The listing builds one solid part. Answer for the finished solid, in the listing's coordinates (mm). A direction names the side the tool comes from. Round coordinates to 2 decimals unless told otherwise and drop trailing zeros. Order: outer loops, then holes, each group sorted by start corner. A loop starts at its lowest first (then second) coordinate and runs counter-clockwise, first axis right, second up. Notation, with made-up numbers: (26, 59.5) -> (46, 59.5) arc R15 cw to (46, 69.5) -> close; hole circle Ø9 at (57.25, -11.5). An arc over 180 degrees is marked (long way). Answer in a Markdown table with one row per item. Add a question column.
Solid Edge part; units mm, degrees
sketch "Sketch1" plane through (0, 0, 0) normal (0, 0, 1) x (1, 0, 0)
  line L0 (0, 32.5628) -> (110, 32.5628)
  line L1 (110, 32.5628) -> (110, -77.4372)
  line L2 (110, -77.4372) -> (0, -77.4372)
  line L3 (0, 32.5628) -> (0, -77.4372)
extrude "Protrusion1" add sketch "Sketch1" along normal blind 27
sketch "Sketch2" plane through (55, -22.4372, 27) normal (0, 0, 1) x (1, 0, 0)
  line L0 (-53, -53) -> (53, -53)
  line L1 (53, -53) -> (53, 53)
  line L2 (53, 53) -> (-53, 53)
  line L3 (-53, 53) -> (-53, -53)
extrude "ExtrudedCutout_1" cut sketch "Sketch2" against normal blind 25
sketch "Sketch3" plane through (55, 30.5628, 14.5) normal (0, -1, 0) x (1, 0, 0)
  circle A0 centre (-18.3168, -3.0528) radius 6
extrude "ExtrudedCutout_2" cut sketch "Sketch3" against normal blind 2
sketch "Sketch4" plane through (110, -22.4372, 13.5) normal (1, 0, 0) x (0, 1, 0)
  line L0 (23.663, -1.8749) -> (45.663, -1.8749)
  line L1 (45.663, -1.8749) -> (45.663, 3.8251)
  line L2 (45.663, 3.8251) -> (23.663, 3.8251)
  line L3 (23.663, 3.8251) -> (23.663, -1.8749)
extrude "ExtrudedCutout_3" cut sketch "Sketch4" against normal blind 2
sketch "Sketch5" plane through (108, -22.4372, 14.5) normal (-1, 0, 0) x (0, 0, 1)
  line L0 (2.8251, 47.663) -> (4.8251, 47.663)
  line L1 (4.8251, 47.663) -> (4.8251, 21.663)
  line L2 (4.8251, 21.663) -> (-4.8749, 21.663)
  line L3 (-4.8749, 21.663) -> (-4.8749, 47.663)
  line L4 (-4.8749, 47.663) -> (2.8251, 47.663)
extrude "ExtrudedProtrusion_2" add sketch "Sketch5" along normal blind 7.2
sketch "Sketch6" plane through (110, -22.4372, 13.5) normal (1, 0, 0) x (0, 1, 0)
  line L0 (23.663, 3.8251) -> (45.663, 3.8251)
  line L1 (45.663, 3.8251) -> (45.663, -1.8749)
  line L2 (45.663, -1.8749) -> (23.663, -1.8749)
  line L3 (23.663, -1.8749) -> (23.663, 3.8251)
extrude "ExtrudedCutout_4" cut sketch "Sketch6" against normal blind 7
sketch "Sketch7" plane through (100.8, 12.2258, 14.4751) normal (-1, 0, 0) x (0, -1, 0)
  line L0 (0, -1.85) -> (9, -1.85)
  line L1 (9, -1.85) -> (9, 1.85)
  line L2 (9, 1.85) -> (-9, 1.85)
  line L3 (-9, 1.85) -> (-9, -1.85)
  line L4 (-9, -1.85) -> (0, -1.85)
extrude "ExtrudedCutout_5" cut sketch "Sketch7" against normal blind 26.8721
sketch "Sketch8" plane through (110, -22.4372, 13.5) normal (1, 0, 0) x (0, 1, 0)
  line L0 (8.2756, -1.8749) -> (17.2756, -1.8749)
  line L1 (17.2756, -1.8749) -> (17.2756, 3.8251)
  line L2 (17.2756, 3.8251) -> (8.2756, 3.8251)
  line L3 (8.2756, 3.8251) -> (8.2756, -1.8749)
extrude "ExtrudedCutout_6" cut sketch "Sketch8" against normal blind 30.5101
sketch "Sketch9" plane through (108, -22.4372, 14.5) normal (-1, 0, 0) x (0, -1, 0)
  line L0 (-17.2756, 4.8251) -> (-6.2756, 4.8251)
  line L1 (-6.2756, 4.8251) -> (-6.2756, -4.8749)
  line L2 (-6.2756, -4.8749) -> (-19.2756, -4.8749)
  line L3 (-19.2756, -4.8749) -> (-19.2756, 4.8251)
  line L4 (-19.2756, 4.8251) -> (-17.2756, 4.8251)
extrude "ExtrudedProtrusion_3" add sketch "Sketch9" along normal blind 7.2
sketch "Sketch10" plane through (108, -9.6616, 14.4751) normal (1, 0, 0) x (0, 1, 0)
  line L0 (-2.5, -1.85) -> (0, -1.85)
  line L1 (0, -1.85) -> (2.5, -1.85)
  line L2 (2.5, -1.85) -> (2.5, 1.85)
  line L3 (2.5, 1.85) -> (-2.5, 1.85)
  line L4 (-2.5, 1.85) -> (-2.5, -1.85)
extrude "ExtrudedCutout_8" cut sketch "Sketch10" against normal blind 9.4627
sketch "Sketch11" plane through (108, -9.6616, 14.4751) normal (1, 0, 0) x (0, 1, 0)
  line L0 (-4.5, 2.85) -> (4.5, 2.85)
  line L1 (4.5, 2.85) -> (4.5, -2.85)
  line L2 (4.5, -2.85) -> (-4.5, -2.85)
  line L3 (-4.5, -2.85) -> (-4.5, 2.85)
extrude "ExtrudedCutout_10" cut sketch "Sketch11" against normal blind 7
sketch "Sketch12" plane through (0, -22.4372, 13.5) normal (-1, 0, 0) x (0, -1, 0)
  line L0 (-45.663, 3.8251) -> (-45.663, -1.8749)
  line L1 (-45.663, -1.8749) -> (-25.663, -1.8749)
  line L2 (-25.663, -1.8749) -> (-25.663, 3.8251)
  line L3 (-25.663, 3.8251) -> (-45.663, 3.8251)
extrude "ExtrudedCutout_11" cut sketch "Sketch12" against normal blind 2
sketch "Sketch13" plane through (2, -22.4372, 14.5) normal (1, 0, 0) x (0, 0, -1)
  line L0 (4.8749, 23.663) -> (-4.8251, 23.663)
  line L1 (-4.8251, 23.663) -> (-4.8251, 47.663)
  line L2 (-4.8251, 47.663) -> (4.8749, 47.663)
  line L3 (4.8749, 47.663) -> (4.8749, 23.663)
extrude "ExtrudedProtrusion_4" add sketch "Sketch13" along normal blind 7.2
sketch "Sketch14" plane through (0, -22.4372, 13.5) normal (-1, 0, 0) x (0, -1, 0)
  line L0 (-45.663, -1.8749) -> (-45.663, 3.8251)
  line L1 (-45.663, 3.8251) -> (-25.663, 3.8251)
  line L2 (-25.663, 3.8251) -> (-25.663, -1.8749)
  line L3 (-25.663, -1.8749) -> (-45.663, -1.8749)
extrude "ExtrudedCutout_12" cut sketch "Sketch14" against normal blind 7
sketch "Sketch15" plane through (7, 13.2258, 14.4751) normal (-1, 0, 0) x (0, 0, 1)
  line L0 (1.85, 8) -> (-1.85, 8)
  line L1 (-1.85, 8) -> (-1.85, -8)
  line L2 (-1.85, -8) -> (1.85, -8)
  line L3 (1.85, -8) -> (1.85, 8)
extrude "Cutout1" cut sketch "Sketch15" against normal blind 13.8716
sketch "Sketch16" plane through (2, -22.4372, 14.5) normal (1, 0, 0) x (0, 0, -1)
  line L0 (-4.8251, 19.2756) -> (4.8749, 19.2756)
  line L1 (4.8749, 19.2756) -> (4.8749, 6.2756)
  line L2 (4.8749, 6.2756) -> (-4.8251, 6.2756)
  line L3 (-4.8251, 6.2756) -> (-4.8251, 19.2756)
extrude "ExtrudedProtrusion_7" add sketch "Sketch16" along normal blind 7.2
sketch "Sketch17" plane through (9.2, -9.6616, 14.4751) normal (1, 0, 0) x (0, 0, -1)
  line L0 (-1.85, 2.5) -> (1.85, 2.5)
  line L1 (1.85, 2.5) -> (1.85, -2.5)
  line L2 (1.85, -2.5) -> (-1.85, -2.5)
  line L3 (-1.85, -2.5) -> (-1.85, 2.5)
extrude "ExtrudedCutout_16" cut sketch "Sketch17" against normal blind 15.454
sketch "Sketch18" plane through (0, -22.4372, 13.5) normal (-1, 0, 0) x (0, 0, 1)
  line L0 (-1.8749, 17.2756) -> (3.8251, 17.2756)
  line L1 (3.8251, 17.2756) -> (3.8251, 8.2756)
  line L2 (3.8251, 8.2756) -> (-1.8749, 8.2756)
  line L3 (-1.8749, 8.2756) -> (-1.8749, 17.2756)
extrude "ExtrudedCutout_17" cut sketch "Sketch18" against normal blind 7
sketch "Sketch19" plane through (2, -22.4372, 14.5) normal (1, 0, 0) x (0, 0, -1)
  line L0 (-4.8251, 1.8941) -> (4.8749, 1.8941)
  line L1 (4.8749, 1.8941) -> (4.8749, -11.1059)
  line L2 (4.8749, -11.1059) -> (-4.8251, -11.1059)
  line L3 (-4.8251, -11.1059) -> (-4.8251, 1.8941)
extrude "ExtrudedProtrusion_8" add sketch "Sketch19" along normal blind 7.2
sketch "Sketch20" plane through (9.2, -27.0431, 14.4751) normal (1, 0, 0) x (0, 0, -1)
  line L0 (-1.85, 2.5) -> (-1.85, -2.5)
  line L1 (-1.85, -2.5) -> (1.85, -2.5)
  line L2 (1.85, -2.5) -> (1.85, 2.5)
  line L3 (1.85, 2.5) -> (-1.85, 2.5)
extrude "ExtrudedCutout_18" cut sketch "Sketch20" against normal blind 324.0976
sketch "Sketch21" plane through (0, -22.4372, 13.5) normal (-1, 0, 0) x (0, 0, 1)
  line L0 (-1.8749, -0.1059) -> (3.8251, -0.1059)
  line L1 (3.8251, -0.1059) -> (3.8251, -9.1059)
  line L2 (3.8251, -9.1059) -> (-1.8749, -9.1059)
  line L3 (-1.8749, -9.1059) -> (-1.8749, -0.1059)
extrude "ExtrudedCutout_19" cut sketch "Sketch21" against normal blind 7
sketch "Sketch22" plane through (55, -22.4372, 27) normal (0, 0, 1) x (1, 0, 0)
  line L0 (-55, 55) -> (55, 55)
  line L1 (55, 55) -> (55, -55)
  line L2 (55, -55) -> (-55, -55)
  line L3 (-55, -55) -> (-55, 55)
extrude "ExtrudedProtrusion_9" add sketch "Sketch22" along normal blind 35
sketch "Sketch23" plane through (55, -22.4372, 62) normal (0, 0, 1) x (1, 0, 0)
  line L0 (-53, 53) -> (53, 53)
  line L1 (53, 53) -> (53, -53)
  line L2 (53, -53) -> (-53, -53)
  line L3 (-53, -53) -> (-53, 53)
extrude "Cutout2" cut sketch "Sketch23" against normal blind 35
sketch "Sketch24" plane through (55, -22.4372, 62) normal (0, 0, 1) x (1, 0, 0)
  line L0 (-55, 55) -> (55, 55)
  line L1 (55, 55) -> (55, -55)
  line L2 (55, -55) -> (-55, -55)
  line L3 (-55, -55) -> (-55, 55)
extrude "ExtrudedCutout_21" cut sketch "Sketch24" against normal blind 18
sketch "Sketch25" plane through (55, -22.4372, 0) normal (0, 0, -1) x (-1, 0, 0)
  line L0 (-55, 55) -> (55, 55)
  line L1 (55, 55) -> (55, -55)
  line L2 (55, -55) -> (-55, -55)
  line L3 (-55, -55) -> (-55, 55)
extrude "Protrusion2" add sketch "Sketch25" along normal blind 17
sketch "Sketch26" plane through (55, -22.4372, 2) normal (0, 0, 1) x (-1, 0, 0)
  line L0 (-53, 53) -> (53, 53)
  line L1 (53, 53) -> (53, -53)
  line L2 (53, -53) -> (-53, -53)
  line L3 (-53, -53) -> (-53, 53)
extrude "ExtrudedCutout_22" cut sketch "Sketch26" against normal blind 17
1. The part is cut by section D-D (y = 9). Give the number of separate pieces and of enclosed holes in the cut face, then the cut area to 3 significant figures.
2. The mould has two halves that part along Y. Classify faces 4 (the flat face through (104, -0.774, 15)), 5 (the flat face through (54, 32.563, 13)), 6 (the flat face through (107, 1.226, 15)), 7 (the flat face through (110, -22, 13)): released by +Y, released by -Y, zero draft, split by the parting line, or undercut.
3. The part is cut by section B-B (z = 21). Give the vertices of the cut face in (x, y), then the cut area to 3 significant figures.
4. For faces 1 (the flat face through (9.2, -10, 17)), 2 (the flat face through (7, 13, 12)), 3 (the flat face through (104, -10, 9.625)), determine the directions among +Z, -Z, +X, -X, +Y, -Y from which every point of the face is accessible in a straight line to the end or side of a thin tool.
5. Each of these flat-tipped pins is pushed along its axis until it touches: pin 1 (4.5 mm diameter, centred on y = -26.5, z = 15.5, fed in from -X); pin 2 (3 mm diameter, centred on y = -7.5, z = 14, fed in from -X); pin 3 (5 mm diameter, centred on x = 31, y = -40, fed in from +Z); pin 4 (8 mm diameter, centred on x = 7, y = 12, fed in from +Z). Where does it stop, or does it pass through?
6. The part is cut by section A-A (y = -26). Give the vertices of the cut face in (x, z).
7. The part is cut by section C-C (x = 58). Give the vertices of the cut face in (y, z).
8. Straight lines are drawn through the part: line 1 along X through (y, z) = (-62.5, 17); line 2 along Y through (x, z) = (60, 8); line 3 along X through (y, z) = (7, 12). For each, find the intervals that lie inside material, in ascending order.
Report:
| question | item | result |
|---|---|---|
| 1 | separate pieces | 3 |
| 1 | enclosed holes | 0 |
| 1 | area | 500 mm^2 |
| 2 | face 4 | undercut |
| 2 | face 5 | released by +Y |
| 2 | face 6 | undercut |
| 2 | face 7 | zero draft |
| 3 | outline | (0, -77.44) -> (110, -77.44) -> (110, 32.56) -> (0, 32.56) -> close; hole (2, -75.44) -> (108, -75.44) -> (108, 30.56) -> (2, 30.56) -> close |
| 3 | area | 864 mm^2 |
| 4 | face 1 | +Z |
| 4 | face 2 | -X |
| 4 | face 3 | none |
| 5 | pin 1 | stops at x = 0 |
| 5 | pin 2 | stops at x = 7 |
| 5 | pin 3 | stops at z = -15 |
| 5 | pin 4 | stops at z = 19.33 |
| 6 | outline | (0, -17) -> (110, -17) -> (110, 44) -> (108, 44) -> (108, -15) -> (2, -15) -> (2, 9.63) -> (9.2, 9.63) -> (9.2, 12.63) -> (7, 12.63) -> (7, 11.63) -> (0, 11.63) -> close; (0, 17.33) -> (7, 17.33) -> (7, 16.33) -> (9.2, 16.33) -> (9.2, 19.33) -> (2, 19.33) -> (2, 44) -> (0, 44) -> close |
| 7 | outline | (-77.44, -17) -> (32.56, -17) -> (32.56, 44) -> (30.56, 44) -> (30.56, -15) -> (-75.44, -15) -> (-75.44, 44) -> (-77.44, 44) -> close |
| 8 | line 1 | x = 0 to 2, 108 to 110 |
| 8 | line 2 | y = -77.44 to -75.44, 30.56 to 32.56 |
| 8 | line 3 | x = 7 to 9.2, 100.8 to 103 |
